from build123d import *

# Parameters (mm, degrees)
SKETCH1_R           = 25.4
SKETCH1_R_2         = 3.175
BOSS_EXTRUDE1_DEPTH = 3.175
ATTACHMENTHOLES_R   = 1.697640298
ATTACHMENTHOLES_R_2 = 1.839394333
ATTACHMENTHOLES_R_3 = 1.494089935
CUT_EXTRUDE1_DEPTH  = 37.061067996


with BuildPart() as part:
    # Sketch1 → Boss-Extrude1 (new body)
    with BuildSketch(Plane.XY):
        Circle(SKETCH1_R)
        Circle(SKETCH1_R_2, mode=Mode.SUBTRACT)
    extrude(amount=BOSS_EXTRUDE1_DEPTH)

    # AttachmentHoles → Cut-Extrude1 (cut, through all)
    with BuildSketch(Plane.XY):
        with Locations((-9.118891252, 6.145879466)):
            Circle(ATTACHMENTHOLES_R)
        with Locations((9.347171253, 3.791989153)):
            Circle(ATTACHMENTHOLES_R_2)
        with Locations((-2.113411396, -11.140283228)):
            Circle(ATTACHMENTHOLES_R_3)
    extrude(amount=CUT_EXTRUDE1_DEPTH, mode=Mode.SUBTRACT)


solid = part.part
Here's how the part is built. I have some questions about the finished solid (model axes, mm). Round coordinates to 2 decimals unless told otherwise and drop trailing zeros. Write each loop counter-clockwise with the first axis right and the second up, starting at its lowest first coordinate (ties: lowest second). Pieces come first, ordered by that corner, then holes.
1. Will these pins go through, and if not, where does the flat tip stop? pin 1 Ø1.5 at (x, z) = (8.5, 1.5) entering from +Y; pin 2 Ø3 at (x, y) = (9.35, 3.79) entering from -Z; pin 3 Ø1 at (x, z) = (2.5, 2.5) entering from -Y.
2. Suppose I cut it at A-A (y = 0). List the corners of the cut face in (x, z) for me (3 decimals), and give its area (3 significant figures).
3. I need wall thicknesses on L1, parallel to Y at x = -9, z = 2.95; L2, parallel to X at y = -1.5, z = 1.25; L3, parallel to Y at x = 11.5, z = 2. Which ranges of each line are inside material? Lowest first, please.
4. If we mould it in two halves opening along Y, with no side actions, what happens to faces 1 (the cylindrical face through (-9.34, 7.83, 1.57)), 2 (the flat face through (5, 0, 0)), 3 (the cylindrical face through (-5.506, -24.796, 1.565))? For each: released by +Y, released by -Y, zero draft, split by the parting line, or undercut.
5. Suppose I cut it at D-D (x = 21). List the corners of the cut face in (y, z) for me (3 decimals).
6. Suppose I cut it at B-B (x = -9.5). List the corners of the cut face in (y, z) for me (3 decimals).
7. Suppose I cut it at C-C (z = 2.6). List the corners of the cut face in (x, y) for me (3 decimals), and give its area (3 significant figures).
Answer sheet:
1. pin 1: stops at y = 24.19
1. pin 2: passes through
1. pin 3: stops at y = -25.32
2. outline: (-25.4, 0) - (-3.175, 0) - (-3.175, 3.175) - (-25.4, 3.175) - close; (3.175, 0) - (25.4, 0) - (25.4, 3.175) - (3.175, 3.175) - close
2. area: 141 mm2
3. L1: y = -23.75 to 4.45, 7.84 to 23.75
3. L2: x = -25.36 to -2.8, 2.8 to 25.36
3. L3: y = -22.65 to 22.65
4. face 1: undercut
4. face 2: zero draft
4. face 3: split by the parting line
5. outline: (-14.288, 0) - (14.288, 0) - (14.288, 3.175) - (-14.288, 3.175) - close
6. outline: (-23.557, 0) - (4.492, 0) - (4.492, 3.175) - (-23.557, 3.175) - close; (7.8, 0) - (23.557, 0) - (23.557, 3.175) - (7.8, 3.175) - close
7. outline: circle Ø50.8 at (0, 0); hole circle Ø3.395 at (-9.119, 6.146); hole circle Ø2.988 at (-2.113, -11.14); hole circle Ø6.35 at (0, 0); hole circle Ø3.679 at (9.347, 3.792)
7. area: 1,970 mm2
